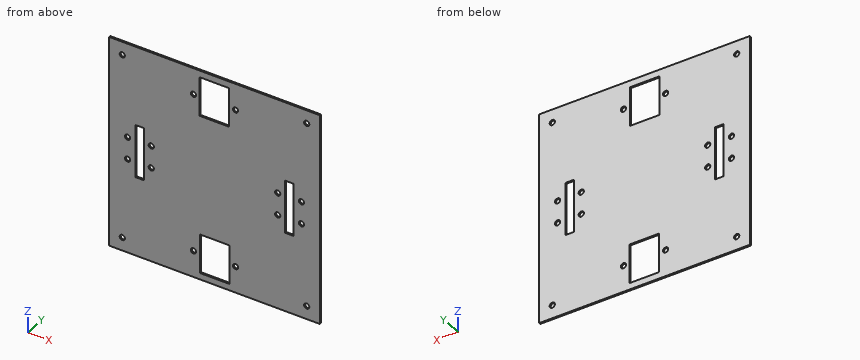
```python
from build123d import *

# Parameters (mm, degrees)
SKETCH1_W           = 400
SKETCH1_H           = 400
BOSS_EXTRUDE1_DEPTH = 3
SKETCH3_W           = 16
SKETCH3_H           = 100
CUT_EXTRUDE1_DEPTH  = 3
SKETCH4_W           = 56
SKETCH4_H           = 74
CUT_EXTRUDE2_DEPTH  = 3
SKETCH5_R           = 5
CUT_EXTRUDE3_DEPTH  = 3


with BuildPart() as part:
    # Sketch1 → Boss-Extrude1 (new body)
    with BuildSketch(Plane(origin=(0, 0, 0), x_dir=(1, 0, 0), z_dir=(0, 1, 0))):
        Rectangle(SKETCH1_W, SKETCH1_H)
    extrude(amount=BOSS_EXTRUDE1_DEPTH)

    # Sketch3 → Cut-Extrude1 (cut)
    with BuildSketch(Plane(origin=(0, 3, 0), x_dir=(1, 0, 0), z_dir=(0, 1, 0))):
        with Locations((-141.990723633, 0.005834667)):
            Rectangle(SKETCH3_W, SKETCH3_H)
        with Locations((141.996469981, 0.005657447)):
            Rectangle(SKETCH3_W, SKETCH3_H)
    extrude(amount=-CUT_EXTRUDE1_DEPTH, mode=Mode.SUBTRACT)

    # Sketch4 → Cut-Extrude2 (cut)
    with BuildSketch(Plane(origin=(0, 3, 0), x_dir=(1, 0, 0), z_dir=(0, 1, 0))):
        with Locations((0.607935106, 150.770035388)):
            Rectangle(SKETCH4_W, SKETCH4_H)
        with Locations((-0.434902884, -150.241190723)):
            Rectangle(SKETCH4_W, SKETCH4_H)
    extrude(amount=-CUT_EXTRUDE2_DEPTH, mode=Mode.SUBTRACT)

    # Sketch5 → Cut-Extrude3 (cut)
    with BuildSketch(Plane(origin=(0, 3, 0), x_dir=(1, 0, 0), z_dir=(0, 1, 0))):
        with Locations(Location((-165, 21, 0), (0, 0, 270))):
            Circle(SKETCH5_R)
        with Locations(Location((-165, -21, 0), (0, 0, 270))):
            Circle(SKETCH5_R)
        with Locations(Location((-120, 21, 0), (0, 0, 270))):
            Circle(SKETCH5_R)
        with Locations(Location((-120, -21, 0), (0, 0, 270))):
            Circle(SKETCH5_R)
        with Locations(Location((165, 21, 0), (0, 0, 270))):
            Circle(SKETCH5_R)
        with Locations(Location((165, -21, 0), (0, 0, 270))):
            Circle(SKETCH5_R)
        with Locations(Location((120, 21, 0), (0, 0, 270))):
            Circle(SKETCH5_R)
        with Locations(Location((120, -21, 0), (0, 0, 270))):
            Circle(SKETCH5_R)
        with Locations(Location((-40, -150, 0), (0, 0, 270))):
            Circle(SKETCH5_R)
        with Locations(Location((40, -150, 0), (0, 0, 270))):
            Circle(SKETCH5_R)
        with Locations(Location((-40, 150, 0), (0, 0, 270))):
            Circle(SKETCH5_R)
        with Locations(Location((40, 150, 0), (0, 0, 270))):
            Circle(SKETCH5_R)
        with Locations(Location((-175, 175, 0), (0, 0, 270))):
            Circle(SKETCH5_R)
        with Locations(Location((175, 175, 0), (0, 0, 270))):
            Circle(SKETCH5_R)
        with Locations(Location((175, -175, 0), (0, 0, 270))):
            Circle(SKETCH5_R)
        with Locations(Location((-175, -175, 0), (0, 0, 270))):
            Circle(SKETCH5_R)
    extrude(amount=-CUT_EXTRUDE3_DEPTH, mode=Mode.SUBTRACT)


solid = part.part
```
Input: part model. Units: mm. Frame: model coordinates. Coordinates: 2 decimals unless noted, no trailing zeros. Loops run counter-clockwise (first coordinate to the right, second up) from the corner with the lowest first, then second, coordinate; pieces in that order, holes last. Notation, with made-up numbers: (49, -24.75) - (70, -24.75) arc R17 ccw to (70, -19.75) - close; hole circle Ø2 at (56, -9.75). An arc over 180 degrees is marked (long way). Answer in a Markdown table with one row per item.
(1) Material intervals for L1, parallel to X at y = 1, z = 150; L2, parallel to X at y = 0.7, z = -150; L3, parallel to X at y = 0.9, z = -31.5, sorted ascending. Write a range as from..to.
Model answer:
| item | result |
|---|---|
| L1 | x = -200..-45, -35..-28.43, 27.57..35, 45..200 |
| L2 | x = -200..-45, -35..-27.39, 28.61..35, 45..200 |
| L3 | x = -200..-149.99, -133.99..134, 150..200 |
(2) Cut plane D-D on z = -120.5. Output: boundary loops of the cut face in (x, y).
Model answer:
| item | result |
|---|---|
| outline | (-200, 0) - (-27.39, 0) - (-27.39, 3) - (-200, 3) - close; (28.61, 0) - (200, 0) - (200, 3) - (28.61, 3) - close |
(3) Cut plane A-A on z = 21. Output: boundary loops of the cut face in (x, y), plus the area to 3 significant figures.
Model answer:
| item | result |
|---|---|
| outline | (-200, 0) - (-170, 0) - (-170, 3) - (-200, 3) - close; (-160, 0) - (-149.99, 0) - (-149.99, 3) - (-160, 3) - close; (-133.99, 0) - (-125, 0) - (-125, 3) - (-133.99, 3) - close; (-115, 0) - (115, 0) - (115, 3) - (-115, 3) - close; (125, 0) - (134, 0) - (134, 3) - (125, 3) - close; (150, 0) - (160, 0) - (160, 3) - (150, 3) - close; (170, 0) - (200, 0) - (200, 3) - (170, 3) - close |
| area | 984 mm² |
(4) Cut plane B-B on x = 4.5. Output: boundary loops of the cut face in (y, z).
Model answer:
| item | result |
|---|---|
| outline | (0, -200) - (3, -200) - (3, -187.77) - (0, -187.77) - close; (0, -113.77) - (3, -113.77) - (3, 113.24) - (0, 113.24) - close; (0, 187.24) - (3, 187.24) - (3, 200) - (0, 200) - close |
(5) Cut plane C-C on z = 175. Output: boundary loops of the cut face in (x, y).
Model answer:
| item | result |
|---|---|
| outline | (-200, 0) - (-180, 0) - (-180, 3) - (-200, 3) - close; (-170, 0) - (-28.43, 0) - (-28.43, 3) - (-170, 3) - close; (27.57, 0) - (170, 0) - (170, 3) - (27.57, 3) - close; (180, 0) - (200, 0) - (200, 3) - (180, 3) - close |
